Geometry check sheet. Reference: drawing and pictorial views, mm from the part's lowest x, y, z. Give positions to 0.01 mm unless a question says otherwise; leave off trailing zeros. Order: outer loops, then holes, each group sorted by start corner. A loop starts at its lowest first (then second) coordinate and runs counter-clockwise, first axis right, second up. Notation, with made-up numbers: (52.5, 5.25) -> (109.5, 5.25) arc R29 ccw to (109.5, 36.25) -> close; hole circle Ø6 at (70.5, 78). An arc over 180 degrees is marked (long way). Write each question's results on one line, items separated by ' | '.
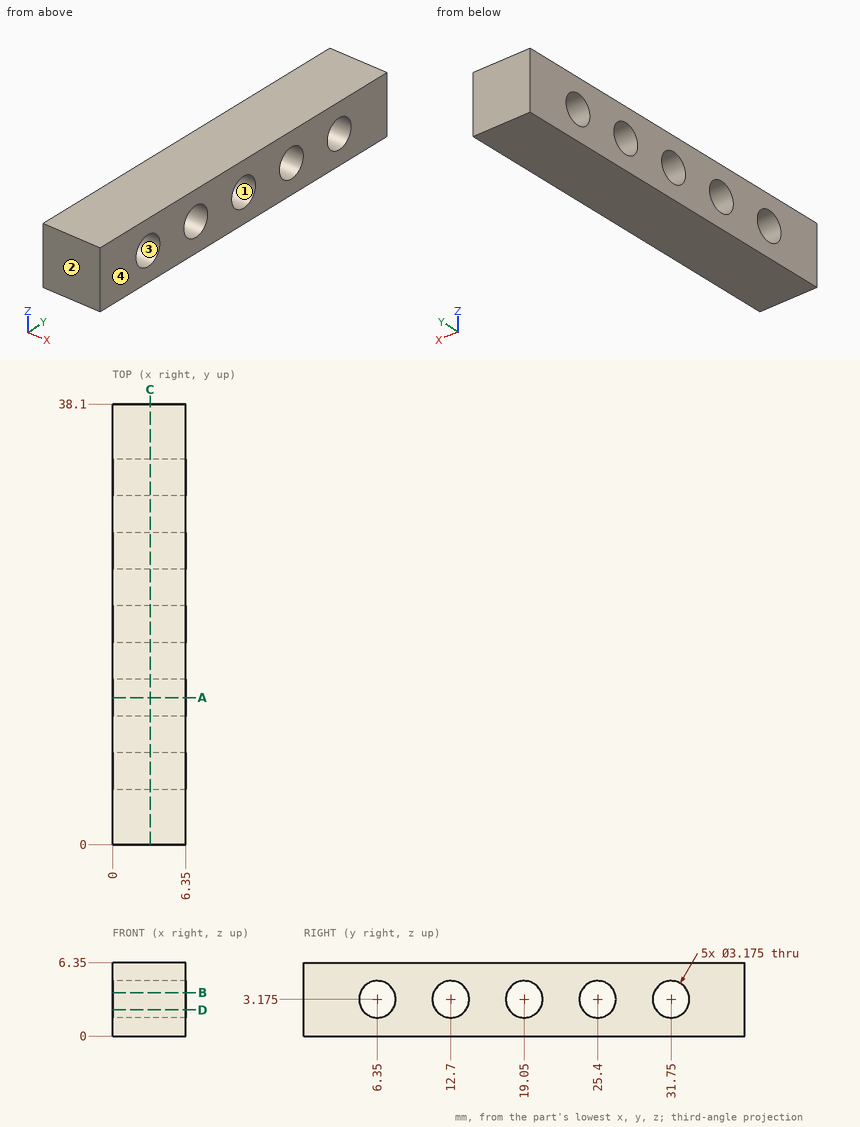
1. Section check C-C on x = 3.25. Give the number of separate pieces and of enclosed holes in the cut face, then the cut area to 3 significant figures.
Verdict:
separate pieces: 1 | enclosed holes: 5 | area: 202 mm^2
2. Mould release check, pull along Y, two halves, no side actions. Record for the marked faces 1, 2, 3 and 4: +Y half, -Y half, draft (parallel to the pull), parting line (faces both ways), or undercut.
Verdict:
face 1: undercut | face 2: -Y half | face 3: undercut | face 4: draft
3. Material ranges on probe 1 along Y at (x, z) = (3.5, 2.5); probe 2 along Y at (x, z) = (4.5, 2.25); probe 3 along Z at (x, y) = (2.25, 25.4), recorded low to high. Write a range as from..to.
Verdict:
probe 1: y = 0..4.91, 7.79..11.26, 14.14..17.61, 20.49..23.96, 26.84..30.31, 33.19..38.1 | probe 2: y = 0..5.06, 7.64..11.41, 13.99..17.76, 20.34..24.11, 26.69..30.46, 33.04..38.1 | probe 3: z = 0..1.59, 4.76..6.35
4. Section check D-D on z = 2.25. Record the cut outline in (x, y).
Verdict:
outline: (0, 0) -> (6.35, 0) -> (6.35, 5.06) -> (0, 5.06) -> close; (0, 7.64) -> (6.35, 7.64) -> (6.35, 11.41) -> (0, 11.41) -> close; (0, 13.99) -> (6.35, 13.99) -> (6.35, 17.76) -> (0, 17.76) -> close; (0, 20.34) -> (6.35, 20.34) -> (6.35, 24.11) -> (0, 24.11) -> close; (0, 26.69) -> (6.35, 26.69) -> (6.35, 30.46) -> (0, 30.46) -> close; (0, 33.04) -> (6.35, 33.04) -> (6.35, 38.1) -> (0, 38.1) -> close
5. Gauge pin test, flat ends, axial feed: pin 1 Ø3 at (y, z) = (31.75, 3.175) entering from -X; pin 2 Ø3.5 at (y, z) = (25.4, 3.175) entering from +X. Record the tip position at first contact, or that the pin passes through.
Verdict:
pin 1: passes through | pin 2: stops at x = 6.35
6. Section check A-A on y = 12.7. Record the cut outline in (x, z).
Verdict:
outline: (0, 0) -> (6.35, 0) -> (6.35, 1.59) -> (0, 1.59) -> close; (0, 4.76) -> (6.35, 4.76) -> (6.35, 6.35) -> (0, 6.35) -> close
7. Section check B-B on z = 3.75. Record the cut outline in (x, y), then the cut area to 3 significant figures.
Verdict:
outline: (0, 0) -> (6.35, 0) -> (6.35, 4.87) -> (0, 4.87) -> close; (0, 7.83) -> (6.35, 7.83) -> (6.35, 11.22) -> (0, 11.22) -> close; (0, 14.18) -> (6.35, 14.18) -> (6.35, 17.57) -> (0, 17.57) -> close; (0, 20.53) -> (6.35, 20.53) -> (6.35, 23.92) -> (0, 23.92) -> close; (0, 26.88) -> (6.35, 26.88) -> (6.35, 30.27) -> (0, 30.27) -> close; (0, 33.23) -> (6.35, 33.23) -> (6.35, 38.1) -> (0, 38.1) -> close | area: 148 mm^2
